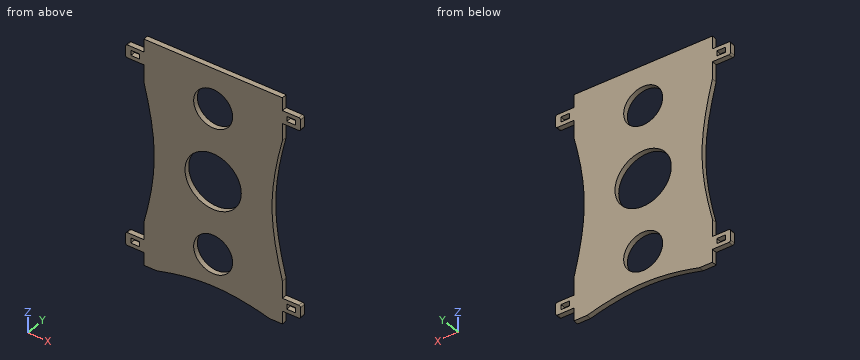
from build123d import *

# Parameters (mm, degrees)
F0_R     = 22.5
F0_R_2   = 32.5
F1_DEPTH = 6
F2_W     = 10
F2_H     = 6
F3_DEPTH = 25
F5_DEPTH = 25


with BuildPart() as f1:
    # F0 (on Front) → F1 (new body)
    with BuildSketch(Plane.XZ):
        Polygon((80, 132), (-80, 132), (-80, 117), (-80, 102), (-80, 74.3303437366), (-80, -102), (-80, -117), (-80, -132), (80, -132), (80, -117), (80, -102), (80, -74.3303437366), (80, 102), (80, 117), align=None)
        with Locations((0, -85)):
            Circle(F0_R, mode=Mode.SUBTRACT)
        Circle(F0_R_2, mode=Mode.SUBTRACT)
        with Locations((0, 85)):
            Circle(F0_R, mode=Mode.SUBTRACT)
        with BuildLine():
            Line((-80, 102), (-80, 117))
            Line((-80, 117), (-99, 117))
            ThreePointArc((-99, 117), (-100.4142135624, 116.4142135624), (-101, 115))
            Line((-101, 115), (-101, 104))
            ThreePointArc((-101, 104), (-100.4142135624, 102.5857864376), (-99, 102))
            Line((-99, 102), (-80, 102))
        make_face()
        with BuildLine():
            Line((99, 117), (80, 117))
            Line((80, 117), (80, 102))
            Line((80, 102), (99, 102))
            ThreePointArc((99, 102), (100.4142135624, 102.5857864376), (101, 104))
            Line((101, 104), (101, 115))
            ThreePointArc((101, 115), (100.4142135624, 116.4142135624), (99, 117))
        make_face()
        with BuildLine():
            Line((-80, -117), (-80, -102))
            Line((-80, -102), (-99, -102))
            ThreePointArc((-99, -102), (-100.4142135624, -102.5857864376), (-101, -104))
            Line((-101, -104), (-101, -115))
            ThreePointArc((-101, -115), (-100.4142135624, -116.4142135624), (-99, -117))
            Line((-99, -117), (-80, -117))
        make_face()
        with BuildLine():
            Line((99, -102), (80, -102))
            Line((80, -102), (80, -117))
            Line((80, -117), (99, -117))
            ThreePointArc((99, -117), (100.4142135624, -116.4142135624), (101, -115))
            Line((101, -115), (101, -104))
            ThreePointArc((101, -104), (100.4142135624, -102.5857864376), (99, -102))
        make_face()
    extrude(amount=F1_DEPTH)

    # F2 (on face) → F3 (cut)
    with BuildSketch(Plane.XZ.offset(6)):
        with Locations((-90, 109.5)):
            Rectangle(F2_W, F2_H)
        with Locations((90, 109.5)):
            Rectangle(F2_W, F2_H)
        with Locations((-90, -109.5)):
            Rectangle(F2_W, F2_H)
        with Locations((90, -109.5)):
            Rectangle(F2_W, F2_H)
    extrude(amount=-F3_DEPTH, mode=Mode.SUBTRACT)

    # F4 (on face) → F5 (cut)
    with BuildSketch(Plane.XZ.offset(6)):
        with BuildLine():
            add(Edge.make_bspline(
                [(-65, -132), (-43.3333333333, -125.837706387), (0, -118.162293613), (43.3333333333, -125.837706387), (65, -132)],
                knots=[0, 0, 0, 0, 0.5, 1, 1, 1, 1], degree=3))
            Line((-65, -132), (-65, -149.1421461105))
            Line((-65, -149.1421461105), (65, -149.1421461105))
            Line((65, -149.1421461105), (65, -132))
        make_face()
        with BuildLine():
            Line((104.2380854487, 82), (80, 82))
            add(Edge.make_bspline(
                [(80, 82), (74, 58), (62, 0), (74, -58), (80, -82)],
                knots=[0, 0, 0, 0, 0.5, 1, 1, 1, 1], degree=3))
            Line((80, -82), (104.2380854487, -82))
            Line((104.2380854487, -82), (104.2380854487, 82))
        make_face()
        with BuildLine():
            add(Edge.make_bspline(
                [(-80, 82), (-74, 58), (-62, 0), (-74, -58), (-80, -82)],
                knots=[0, 0, 0, 0, 0.5, 1, 1, 1, 1], degree=3))
            Line((-80, 82), (-104.2380854487, 82))
            Line((-104.2380854487, 82), (-104.2380854487, -82))
            Line((-104.2380854487, -82), (-80, -82))
        make_face()
    extrude(amount=-F5_DEPTH, mode=Mode.SUBTRACT)


solid = f1.part
Model file for the job. Use its own axes, mm. Give positions to 0.01 mm unless a question says otherwise; leave off trailing zeros. Order: outer loops, then holes, each group sorted by start corner. A loop starts at its lowest first (then second) coordinate and runs counter-clockwise, first axis right, second up. Notation, with made-up numbers: M 79,-13.5 L 133,-13.5 A33 cw 133,17.5 Z; hole C 37,73 d11. An arc over 180 degrees is marked long. Write item = value, one per line.
Q1. Drill centre lines: line 1 (Z direction, x = 0, y = -3.85); line 2 (Z direction, x = -9.5, y = -4.5); line 3 (X direction, y = -0.25, z = 10.5). Where is each one in solid material? Low to high. Write a range as [from, to].
Derived:
line_1 = [-122, -107.5], [-62.5, -32.5], [32.5, 62.5], [107.5, 132]
line_2 = [-122.24, -105.4], [-64.6, -31.08], [31.08, 64.6], [105.4, 132]
line_3 = [-68.25, -30.76], [30.76, 68.25]
Q2. Cut at B-B, the plane x = 0. Count the separate pieces of the cut face and the enclosed holes in it, then the cut area to 3 significant figures.
Derived:
separate_pieces = 4
enclosed_holes = 0
area = 594 mm2
Q3. Flat gauge pins, fed straight in: pin 1 (3 mm diameter, centred on x = 90, y = -3, fed in from +Z); pin 2 (1.8 mm diameter, centred on x = 86, y = -2, fed in from -Z); pin 3 (1.8 mm diameter, centred on y = -3.5, z = 93.5, fed in from +X). Where does each tip first touch, or does it go through?
Derived:
pin_1 = 117
pin_2 = -117
pin_3 = 80
Q4. Cut at A-A, the plane z = 85. List the corners of the cut face in (x, y), then the cut area to 3 significant figures.
Derived:
outline = M -80,-6 L -22.5,-6 L -22.5,0 L -80,0 Z; M 22.5,-6 L 80,-6 L 80,0 L 22.5,0 Z
area = 690 mm2
